Check sheet for the modelled part. Datum: model origin and axes. Units: mm. A direction names the side the tool comes from. Round coordinates to 2 decimals unless told otherwise and drop trailing zeros. Order: outer loops, then holes, each group sorted by start corner. A loop starts at its lowest first (then second) coordinate and runs counter-clockwise, first axis right, second up.
Q1. Cross-section at B-B on x = 77.5. Record the cut outline in (y, z), then the cut area to 3 significant figures.
Q2. Cross-section at C-C on x = 42.5. Record the cut outline in (y, z) (3 decimals).
Q3. Depth check by flat-ended pin: P1, Ø3, axis at x = 13, z = -36, coming from the -Y side; P2, Ø3, axis at y = 25, z = -26.5, coming from the +X side; P3, Ø4, axis at x = 72.5, z = -12.5, coming from the +Y side; P4, Ø10, axis at y = 13, z = -38, coming from the +X side. Enter the tip coordinate at first touch or a pass-through.
Q4. Cross-section at D-D on z = 7.5. Record the cut outline in (x, y) (3 decimals), then the cut area to 3 significant figures.
Q5. Mould release check, pull along Z, two halves, no side actions. Record for faces 1 (the flat face through (42, 9, 15)), 2 (the flat face through (74, 10, -14)), 3 (the flat face through (53.625, 22, -36)): +Z half, -Z half, draft (parallel to the pull), parting line (faces both ways), or undercut.
Q6. Set-up check for faces 4 (the cylindrical face through (42.255, 3.878, -35.926)), 5 (the flat face through (0, 4, -14)): record each of +Z, -Z, +X, -X, +Y, -Y from which the full face is reachable in a straight line by a thin tool's end or side.
Q7. Cross-section at A-A on z = -12.5. Record the cut outline in (x, y), then the cut area to 3 significant figures.
Q8. Scan lines: probe 1 along Z at (x, y) = (43, 4.75); probe 2 along X at (y, z) = (4, -12.5); probe 3 along X at (y, z) = (15, 11.95). Record each from-to range of solid material in increasing order.
from build123d import *

# Parameters (mm, degrees)
SKETCH2_R                = 5
BOSS_EXTRUDE1_DEPTH      = 15
BOSS_EXTRUDE1_DEPTH_BACK = 44.5
SKETCH3_R                = 1.6
SKETCH3_R_2              = 1.7
CUT_EXTRUDE1_DEPTH       = 31
CUT_EXTRUDE1_DEPTH_BACK  = 1
FILLET1_R                = 2.5
CUT_EXTRUDE5_START       = 10
CUT_EXTRUDE5_DEPTH       = 7.25
CUT_EXTRUDE6_START       = -39.5
CUT_EXTRUDE6_DEPTH       = 7.25
FILLET2_R                = 2


with BuildPart() as part:
    # Sketch2 → Boss-Extrude1 (new body, two sides)
    with BuildSketch(Plane.XY) as boss_extrude1_sk:
        Polygon((0, 10), (0, 0), (85, 0), (85, 10), (62.5, 10), (62.5, 30), (22.5, 30), (22.5, 10), align=None)
        with Locations((42.5, 15)):
            Circle(SKETCH2_R, mode=Mode.SUBTRACT)
    extrude(amount=BOSS_EXTRUDE1_DEPTH)
    extrude(boss_extrude1_sk.sketch, amount=-BOSS_EXTRUDE1_DEPTH_BACK)

    # Sketch3 → Cut-Extrude1 (cut, two sides)
    with BuildSketch(Plane(origin=(0, 0, 0), x_dir=(1, 0, 0), z_dir=(0, 1, 0))) as cut_extrude1_sk:
        with Locations((72.5, 12.5)):
            Circle(SKETCH3_R)
        with Locations((12.5, 12.5)):
            Circle(SKETCH3_R)
        with Locations((7.5, -7.5)):
            Circle(SKETCH3_R_2)
        with Locations((77.5, -7.5)):
            Circle(SKETCH3_R_2)
        with Locations((12.5, 37.5)):
            Circle(SKETCH3_R_2)
        with Locations((72.5, 37.5)):
            Circle(SKETCH3_R_2)
    extrude(amount=CUT_EXTRUDE1_DEPTH, mode=Mode.SUBTRACT)
    extrude(cut_extrude1_sk.sketch, amount=-CUT_EXTRUDE1_DEPTH_BACK, mode=Mode.SUBTRACT)

    # Fillet1
    fillet1_edges = [part.edges().sort_by_distance(p)[0] for p in [
        (62.5, 30, -14.75),
        (62.5, 10, -14.75),
        (85, 10, -14.75),
        (0, 10, -14.75),
        (22.5, 10, -14.75),
        (22.5, 30, -14.75),
    ]]
    fillet(fillet1_edges, radius=FILLET1_R)

    # Sketch5 → Cut-Extrude5 (cut)
    with BuildSketch(Plane.XY.offset(CUT_EXTRUDE5_START)):
        with BuildLine():
            Line((31.375, 30), (31.375, 15))
            ThreePointArc((31.375, 15), (42.5, 3.875), (53.625, 15))
            Line((53.625, 15), (53.625, 30))
            Line((53.625, 30), (31.375, 30))
        make_face()
    extrude(amount=-CUT_EXTRUDE5_DEPTH, mode=Mode.SUBTRACT)

    # Sketch5<2> → Cut-Extrude6 (cut)
    with BuildSketch(Plane.XY.offset(CUT_EXTRUDE6_START)):
        with BuildLine():
            Line((31.375, 30), (31.375, 15))
            ThreePointArc((31.375, 15), (42.5, 3.875), (53.625, 15))
            Line((53.625, 15), (53.625, 30))
            Line((53.625, 30), (31.375, 30))
        make_face()
    extrude(amount=CUT_EXTRUDE6_DEPTH, mode=Mode.SUBTRACT)

    # Fillet2
    fillet2_edges = [part.edges().sort_by_distance(p)[0] for p in [
        (42.5, 30, 2.75),
        (42.5, 30, 10),
        (42.5, 30, -39.5),
        (42.5, 30, -32.25),
    ]]
    fillet(fillet2_edges, radius=FILLET2_R)


solid = part.part
Results found:
1. outline: (0, -44.5) - (10, -44.5) - (10, 5.8) - (0, 5.8) - close; (0, 9.2) - (10, 9.2) - (10, 15) - (0, 15) - close
1. area: 561 mm2
2. outline: (0, -44.5) - (10, -44.5) - (10, -39.5) - (3.875, -39.5) - (3.875, -32.25) - (10, -32.25) - (10, 2.75) - (3.875, 2.75) - (3.875, 10) - (10, 10) - (10, 15) - (0, 15) - close; (20, -44.5) - (30, -44.5) - (30, -41.5) arc R2 ccw to (28, -39.5) - (20, -39.5) - close; (20, -32.25) - (28, -32.25) arc R2 ccw to (30, -30.25) - (30, 0.75) arc R2 ccw to (28, 2.75) - (20, 2.75) - close; (20, 10) - (28, 10) arc R2 ccw to (30, 12) - (30, 15) - (20, 15) - close
3. P1: stops at y = 0
3. P2: stops at x = 62.5
3. P3: stops at y = 10
3. P4: stops at x = 84.95
4. outline: (0, 0) - (5.8, 0) - (5.8, 10) - (2.5, 10) arc R2.5 ccw to (0, 7.5) - close; (9.2, 0) - (75.8, 0) - (75.8, 10) - (65, 10) arc R2.5 cw to (62.5, 12.5) - (62.5, 27.5) arc R2.5 ccw to (60, 30) - (53.625, 30) - (53.625, 15) arc R11.125 cw to (31.375, 15) - (31.375, 30) - (25, 30) arc R2.5 ccw to (22.5, 27.5) - (22.5, 12.5) arc R2.5 cw to (20, 10) - (9.2, 10) - close; (79.2, 0) - (85, 0) - (85, 7.5) arc R2.5 ccw to (82.5, 10) - (79.2, 10) - close
4. area: 1,050 mm2
5. face 1: +Z half
5. face 2: draft
5. face 3: undercut
6. face 4: +Y
6. face 5: +Z, -Z, -X, +Y, -Y
7. outline: (0, 0) - (10.9, 0) - (10.9, 10) - (2.5, 10) arc R2.5 ccw to (0, 7.5) - close; (14.1, 0) - (70.9, 0) - (70.9, 10) - (65, 10) arc R2.5 cw to (62.5, 12.5) - (62.5, 27.5) arc R2.5 ccw to (60, 30) - (25, 30) arc R2.5 ccw to (22.5, 27.5) - (22.5, 12.5) arc R2.5 cw to (20, 10) - (14.1, 10) - close; (74.1, 0) - (85, 0) - (85, 7.5) arc R2.5 ccw to (82.5, 10) - (74.1, 10) - close; hole circle Ø10 at (42.5, 15)
7. area: 1,500 mm2
8. probe 1: z = -44.5 to -39.5, -32.25 to 2.75, 10 to 15
8. probe 2: x = 0 to 10.9, 14.1 to 70.9, 74.1 to 85
8. probe 3: x = 22.5 to 37.5, 47.5 to 62.5
